Here's the drawing with two shaded views (mm, measured from the low corner). I have some questions. Coordinates: 2 decimals unless noted, no trailing zeros. Loops run counter-clockwise (first coordinate to the right, second up) from the corner with the lowest first, then second, coordinate; pieces in that order, holes last. Notation, with made-up numbers: M 3.5,27.5 L 9.5,27.5 A14 cw 9.5,51.5 Z; hole C 26,61.25 d6. An arc over 180 degrees is marked long. Use one line per item in the form item = value. Start each with the question number.
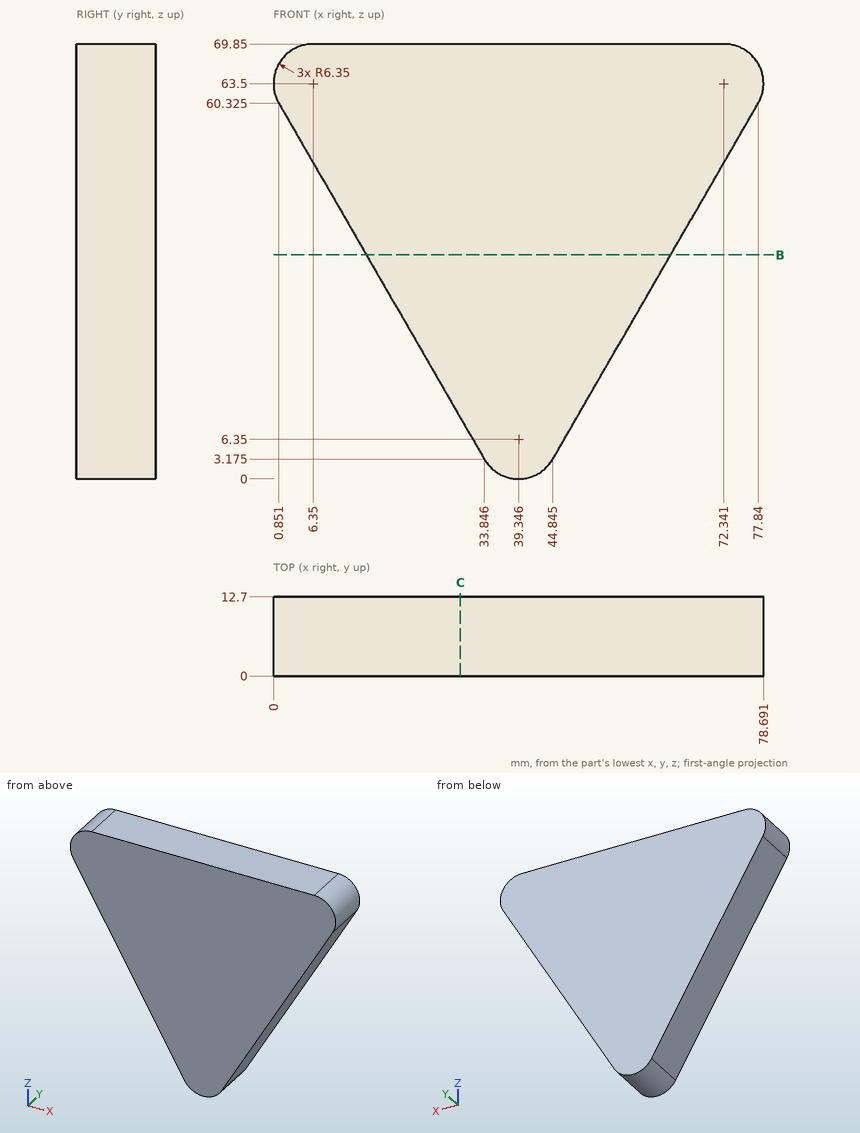
Item 1: Please list where these lines run through material, in increasing order: line 1 along X through (y, z) = (12, 65); line 2 along X through (y, z) = (7, 9.5) (1 decimal); line 3 along Z through (x, y) = (11.5, 12).
Item 2: I want a section at C-C (x = 30). Write out the boundary of the cut face in (y, z).
Item 3: I want a section at B-B (z = 36). Write out the boundary of the cut face in (x, y) (1 decimal), plus the area to 3 significant figures.
Item 4: I'm going to push a flat-ended pin straight in: P1, Ø1.5, axis at y = 3, z = 10.5, coming from the -X side (1 decimal). Where does the tip first touch, or does it pass through?
Worked answers:
q1.line_1 = 0.18 to 78.51
q1.line_2 = 30.2 to 48.5
q1.line_3 = 41.88 to 69.85
q2.outline = M 0,9.84 L 12.7,9.84 L 12.7,69.85 L 0,69.85 Z
q3.outline = M 14.9,0 L 63.8,0 L 63.8,12.7 L 14.9,12.7 Z
q3.area = 621 mm²
q4.P1 = 29.2
